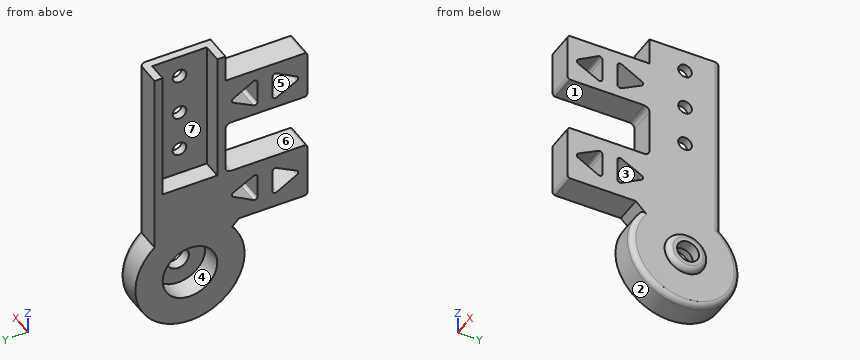
from build123d import *

# Parameters (mm, degrees)
SKETCH_1_R           = 20
SKETCH_1_W           = 63.973509934
SKETCH_1_H           = 26
EXTRUDE_1_DEPTH      = 10
SKETCH_2_W           = 45
SKETCH_2_H           = 20
CUT_EXTRUDE_1_DEPTH  = 7
SKETCH_3_R           = 10
CUT_EXTRUDE_2_DEPTH  = 8
SKETCH_4_R           = 4
CUT_EXTRUDE_3_DEPTH  = 7
SKETCH_6_W           = 10
SKETCH_6_H           = 8
EXTRUDE_2_DEPTH      = 15
CHAMFER_2_SIZE       = 5
EXTRUDE_3_DEPTH      = 20
SKETCH_8_W           = 10
SKETCH_8_H           = 12.77482578
EXTRUDE_4_DEPTH      = 15
SKETCH_9_W           = 7
SKETCH_9_H           = 20
EXTRUDE_5_DEPTH      = 10
SKETCH_10_W          = 7
SKETCH_10_H          = 20
EXTRUDE_6_DEPTH      = 7
SKETCH_11_W          = 10
SKETCH_11_H          = 15
CUT_EXTRUDE_5_DEPTH  = 60.88841868
SKETCH_12_R          = 10
SKETCH_12_W          = 48
SKETCH_12_H          = 20
EXTRUDE_7_DEPTH      = 10
SKETCH_13_R          = 10
CUT_EXTRUDE_6_DEPTH  = 8
SKETCH_14_R          = 4
CUT_EXTRUDE_7_DEPTH  = 8
SKETCH_15_W          = 48
SKETCH_15_H          = 20
CUT_EXTRUDE_8_DEPTH  = 7
SKETCH_16_W          = 10
SKETCH_16_H          = 18
SKETCH_16_H_2        = 20.77482578
EXTRUDE_8_DEPTH      = 15
CUT_EXTRUDE_9_DEPTH  = 15
FILLET_1_R           = 1
FILLET_2_R           = 2
SKETCH_18_R          = 7.5
SKETCH_18_R_2        = 4
EXTRUDE_9_DEPTH      = 2
FILLET_3_R           = 2
SKETCH_19_R          = 2.5
CUT_EXTRUDE_10_DEPTH = 3


# Some blends are built 0.0001 mm under size
with BuildPart() as part:
    # 草图1 → 凸台-拉伸1 (new body)
    with BuildSketch(Plane(origin=(0, 0, 0), x_dir=(0, 0, -1), z_dir=(1, 0, 0))):
        with Locations((31.986754967, 0)):
            Circle(SKETCH_1_R)
        Rectangle(SKETCH_1_W, SKETCH_1_H)
    extrude(amount=EXTRUDE_1_DEPTH)

    # 草图2 → 切除-拉伸1 (cut)
    with BuildSketch(Plane(origin=(10, 0, 0), x_dir=(0, 0, -1), z_dir=(1, 0, 0))):
        with Locations((-9.486754967, 0)):
            Rectangle(SKETCH_2_W, SKETCH_2_H)
    extrude(amount=-CUT_EXTRUDE_1_DEPTH, mode=Mode.SUBTRACT)

    # 草图3 → 切除-拉伸2 (cut)
    with BuildSketch(Plane(origin=(10, 0, 0), x_dir=(0, 0, -1), z_dir=(1, 0, 0))):
        with Locations((31.986754967, 0)):
            Circle(SKETCH_3_R)
    extrude(amount=-CUT_EXTRUDE_2_DEPTH, mode=Mode.SUBTRACT)

    # 草图4 → 切除-拉伸3 (cut)
    with BuildSketch(Plane(origin=(2, 0, 0), x_dir=(0, 0, -1), z_dir=(1, 0, 0))):
        with Locations((31.986754967, 0)):
            Circle(SKETCH_4_R)
    extrude(amount=-CUT_EXTRUDE_3_DEPTH, mode=Mode.SUBTRACT)

    # 草图6 → 凸台-拉伸2 (add)
    with BuildSketch(Plane.XZ.offset(13)):
        with Locations((5, -12.788070813)):
            Rectangle(SKETCH_6_W, SKETCH_6_H)
        with Locations((5, 27.986754967)):
            Rectangle(SKETCH_6_W, SKETCH_6_H)
    extrude(amount=EXTRUDE_2_DEPTH)

    # 倒角2
    # the kernel refuses this chamfer: 5, 3.546264764 mm, written as the material it adds along each edge
    with BuildSketch(Plane(origin=(10, -13, -16.788070813), x_dir=(0, -0.6995038411281902, -0.7146288381019251), z_dir=(-1, 0, 0))) as chamfer_2_piece_1:
        with BuildLine():
            Line((3.535736125, 0), (CHAMFER_2_SIZE * 0.699503841128, CHAMFER_2_SIZE * 0.714628838102))
            Line((CHAMFER_2_SIZE * 0.699503841128, CHAMFER_2_SIZE * 0.714628838102), (0, 0))
            ThreePointArc((0, 0), (1.768947181, 0.07828713), (3.535736125, 0))
        make_face()
    extrude(amount=10)

    # 草图7 → 凸台-拉伸3 (add)
    with BuildSketch(Plane.XY.offset(31.986754967)):
        Polygon((3, -10), (3, 10), (10, 10), (10, 13), (0, 13), (0, -28), (10, -28), (10, -10), align=None)
    extrude(amount=EXTRUDE_3_DEPTH)

    # 草图8 → 凸台-拉伸4 (add)
    with BuildSketch(Plane.XZ.offset(13)):
        with Locations((5, -2.400657923)):
            Rectangle(SKETCH_8_W, SKETCH_8_H)
    extrude(amount=EXTRUDE_4_DEPTH)

    # 草图9 → 凸台-拉伸5 (add)
    with BuildSketch(Plane.XY.offset(-13.013245033)):
        with Locations((6.5, 0)):
            Rectangle(SKETCH_9_W, SKETCH_9_H)
    extrude(amount=EXTRUDE_5_DEPTH)

    # 草图10 → 凸台-拉伸6 (add)
    with BuildSketch(Plane.XY.offset(-3.013245033)):
        with Locations((6.5, 0)):
            Rectangle(SKETCH_10_W, SKETCH_10_H)
    extrude(amount=EXTRUDE_6_DEPTH)

    # 草图11 → 切除-拉伸5 (cut, through all)
    with BuildSketch(Plane(origin=(10, 0, 0), x_dir=(0, 0, -1), z_dir=(1, 0, 0))):
        with Locations((-46.986754967, -20.5)):
            Rectangle(SKETCH_11_W, SKETCH_11_H)
    extrude(amount=-CUT_EXTRUDE_5_DEPTH, mode=Mode.SUBTRACT)

    # 草图12 → 凸台-拉伸7 (add)
    with BuildSketch(Plane(origin=(10, 0, 0), x_dir=(0, 0, -1), z_dir=(1, 0, 0))):
        with Locations((31.986754967, 0)):
            Circle(SKETCH_12_R)
        with Locations((-27.986754967, 0)):
            Rectangle(SKETCH_12_W, SKETCH_12_H)
    extrude(amount=-EXTRUDE_7_DEPTH)

    # 草图13 → 切除-拉伸6 (cut)
    with BuildSketch(Plane.ZY):
        with Locations((-31.986754967, 0)):
            Circle(SKETCH_13_R)
    extrude(amount=-CUT_EXTRUDE_6_DEPTH, mode=Mode.SUBTRACT)

    # 草图14 → 切除-拉伸7 (cut)
    with BuildSketch(Plane.ZY.offset(-8)):
        with Locations((-31.986754967, 0)):
            Circle(SKETCH_14_R)
    extrude(amount=-CUT_EXTRUDE_7_DEPTH, mode=Mode.SUBTRACT)

    # 草图15 → 切除-拉伸8 (cut)
    with BuildSketch(Plane.ZY):
        with Locations((27.986754967, 0)):
            Rectangle(SKETCH_15_W, SKETCH_15_H)
    extrude(amount=-CUT_EXTRUDE_8_DEPTH, mode=Mode.SUBTRACT)

    # 草图16 → 凸台-拉伸8 (add)
    with BuildSketch(Plane.XZ.offset(28)):
        with Locations((5, 32.986754967)):
            Rectangle(SKETCH_16_W, SKETCH_16_H)
        with Locations((5, -6.400657923)):
            Rectangle(SKETCH_16_W, SKETCH_16_H_2)
    extrude(amount=EXTRUDE_8_DEPTH)

    # 草图17 → 切除-拉伸9 (cut)
    with BuildSketch(Plane.ZY):
        Polygon((-0.590983184, -30.271873826), (-12.170144499, -30.271873826), (-6.199884933, -40.719828065), align=None)
        Polygon((-6.199884933, -14.312910757), (-0.590983184, -24.760864996), (-12.170144499, -24.760864996), align=None)
        Polygon((26.997900492, -24.760864996), (38.577061807, -24.760864996), (32.606802242, -14.312910757), align=None)
        Polygon((32.606802242, -40.719828065), (26.997900492, -30.271873826), (38.577061807, -30.271873826), align=None)
    extrude(amount=-CUT_EXTRUDE_9_DEPTH, mode=Mode.SUBTRACT)

    # 圆角1
    fillet_1_edges = [part.edges().sort_by_distance(p)[0] for p in [
        (5, -43, 41.986754967),
        (5, -43, 23.986754967),
        (5, -43, 3.986754967),
        (5, -43, -16.788070813),
        (5, -30.271873826, 38.577061807),
        (5, -40.719828065, 32.606802242),
        (5, -30.271873826, 26.997900492),
        (5, -24.760864996, 26.997900492),
        (5, -14.312910757, 32.606802242),
        (5, -24.760864996, 38.577061807),
        (5, -24.760864996, -12.170144499),
        (5, -14.312910757, -6.199884933),
        (5, -24.760864996, -0.590983184),
        (5, -30.271873826, -0.590983184),
        (5, -40.719828065, -6.199884933),
        (5, -30.271873826, -12.170144499),
    ]]
    fillet(fillet_1_edges, radius=FILLET_1_R)

    # 圆角2
    fillet_2_edges = [part.edges().sort_by_distance(p)[0] for p in [
        (5, -13, 3.986754967),
        (10, 13, 17.599342077),
        (5, -13, 23.986754967),
        (10, 1.767868063, -51.908467808),
    ]]
    fillet(fillet_2_edges, radius=FILLET_2_R)

    # 草图18 → 凸台-拉伸9 (add)
    with BuildSketch(Plane(origin=(10, 0, 0), x_dir=(0, 0, -1), z_dir=(1, 0, 0))):
        with Locations((31.986754967, 0)):
            Circle(SKETCH_18_R)
        with Locations(Location((31.986754967, 0, 0), (0, 0, 180))):
            Circle(SKETCH_18_R_2, mode=Mode.SUBTRACT)
    extrude(amount=EXTRUDE_9_DEPTH)

    # 圆角3
    fillet_3_edges = [part.edges().sort_by_distance(p)[0] for p in [
        (12, 0, -24.486754967),
    ]]
    fillet(fillet_3_edges, radius=FILLET_3_R - 0.0001)  # a hair under: the kernel refuses the full size

    # 草图19 → 切除-拉伸10 (cut)
    with BuildSketch(Plane.ZY.offset(-7)):
        with Locations((43.986754967, 0)):
            Circle(SKETCH_19_R)
        with Locations((28.986754967, 0)):
            Circle(SKETCH_19_R)
        with Locations((13.986754967, 0)):
            Circle(SKETCH_19_R)
    extrude(amount=-CUT_EXTRUDE_10_DEPTH, mode=Mode.SUBTRACT)


solid = part.part
Design review of the part built by this model. Coordinates are the model's own, in mm. Face numbers are marked on the shaded views. A direction names the side the tool comes from. Coordinates: 2 decimals unless noted, no trailing zeros. Order: outer loops, then holes, each group sorted by start corner. A loop starts at its lowest first (then second) coordinate and runs counter-clockwise, first axis right, second up.
Item 1: Take a section at A-A, the plane y = 0. Count the separate pieces of the cut face and the enclosed holes in it, then the cut area to 3 significant figures.
Item 2: Take a section at B-B, the plane z = 0.5. Write out the cut boundary in (x, y).
Item 3: For the marked faces 4, 5, 6 and 7, list the 3-axis set-ups (+Z, -Z, +X, -X, +Y, -Y) from which the entire face can be reached by the end or side of a thin tool; tool diameter is ignored.
Item 4: For line 1 (Z direction, x = 1.25, y = -27); line 2 (Y direction, x = 2.25, z = 10.5); line 3 (Z direction, x = 9, y = -24), list the stretches that pass through material, from the lowest coordinate up.
Item 5: The part is to be moulded in two halves that separate along Y. For the marked faces 1, 2 and 3, say which applies: pulls with the +Y half, pulls with the -Y half, needs draft (parallel to the pull), parting line crosses it, or undercut.
Item 6: For pin 1 Ø5 at (x, z) = (5.5, 18) entering from -Y; pin 2 Ø1 at (y, z) = (-36, -11) entering from +X; pin 3 Ø5 at (x, y) = (3, -23) entering from -Z; pin 4 Ø7 at (y, z) = (0, -31.99) entering from +X, all flat-tipped, find the tip position at first contact; note any pin that passes through.
The answers:
1. separate pieces: 5
1. enclosed holes: 0
1. area: 494 mm2
2. outline: (0, -43) - (10, -43) - (10, 11) arc R2 ccw to (8, 13) - (0, 13) - close
3. face 4: -X
3. face 5: +X, -X
3. face 6: +X, -X, -Y
3. face 7: +Z, -X
4. line 1: z = -16.79 to 3.99, 23.99 to 41.99
4. line 2: y = -13 to -10, 10 to 13
4. line 3: z = -16.79 to -11.42, -1.29 to 3.99, 23.99 to 27.7, 37.82 to 41.99
5. face 1: needs draft
5. face 2: parting line crosses it
5. face 3: undercut
6. pin 1: stops at y = -13
6. pin 2: stops at x = 10
6. pin 3: stops at z = -16.79
6. pin 4: passes through
